```python
from build123d import *

# Parameters (mm, degrees)
EXTRUDE_1_DEPTH     = 43
SKETCH_2_R          = 1.65
CUT_EXTRUDE_1_DEPTH = 40
EXTRUDE_2_DEPTH     = 43
SKETCH_4_R          = 3.5
CUT_EXTRUDE_2_DEPTH = 15


with BuildPart() as part:
    # 草图1 → 凸台-拉伸1 (new body)
    with BuildSketch(Plane.XY):
        Polygon((0, 0), (7.053079228, 40), (37.053079228, 40), align=None)
    extrude(amount=EXTRUDE_1_DEPTH)

    # 草图2 → 切除-拉伸1 (cut)
    with BuildSketch(Plane(origin=(0, 40, 0), x_dir=(1, 0, 0), z_dir=(0, 1, 0))):
        with Locations(Location((10.053079228, -17, 0), (0, 0, 180))):
            Circle(SKETCH_2_R)
        with Locations(Location((10.053079228, -37, 0), (0, 0, 180))):
            Circle(SKETCH_2_R)
    extrude(amount=-CUT_EXTRUDE_1_DEPTH, mode=Mode.SUBTRACT)

    # 草图3 → 凸台-拉伸2 (add)
    with BuildSketch(Plane.XY.offset(43)):
        Polygon((2.644904711, 15), (-3.355095289, 15), (-3.355095289, 0), (0, 0), align=None)
    extrude(amount=-EXTRUDE_2_DEPTH)

    # 草图4 → 切除-拉伸2 (cut)
    with BuildSketch(Plane.XZ):
        with Locations(Location((10.053079228, 37, 0), (0, 0, 270))):
            Circle(SKETCH_4_R)
        with Locations(Location((10.053079228, 17, 0), (0, 0, 270))):
            Circle(SKETCH_4_R)
    extrude(amount=-CUT_EXTRUDE_2_DEPTH, mode=Mode.SUBTRACT)


solid = part.part
```
Work out the finished part from the listing and answer in its coordinate system (mm). A direction names the side the tool comes from. Coordinates: 2 decimals unless noted, no trailing zeros. Write each loop counter-clockwise with the first axis right and the second up, starting at its lowest first coordinate (ties: lowest second). Pieces come first, ordered by that corner, then holes.
Q1. A cutting plane is placed at A-A, the plane z = 17. Give the vertices of the cut face in (x, y).
Q2. Each of these flat-tipped pins is pushed along its axis until it touches: pin 1 Ø10 at (y, z) = (15, 9) entering from +X; pin 2 Ø8 at (x, z) = (10.05, 37) entering from -Y; pin 3 Ø5.5 at (x, z) = (10.05, 37) entering from -Y. Where does it stop, or does it pass through?
Q3. Which of the six approach directions +Z, -Z, +X, -X, +Y, -Y give full straight-line access (tool end or side, diameter ignored) to faces 4 (the face through (18.786, 20.28, 21.199)), 5 (the face through (6.636, 11.827, 17.759))?
Q4. A cutting plane is placed at D-D, the plane x = -1. Give the vertices of the cut face in (y, z), then the cut area to 3 significant figures.
Q5. Determine the mould class of faces 1 (the face through (0, 15, 22)), 2 (the face through (9, 15, 15)), 3 (the face through (4.82, 27.33, 21.2)) for opening direction X: released by +X, released by -X, zero draft, split by the parting line, or undercut.
Q6. A cutting plane is placed at C-C, the plane z = 12. Give the vertices of the cut face in (x, y), then the cut area to 3 significant figures.
Q7. Find the intervals of material crossed by line 1 (Z direction, x = 8, y = 11); line 2 (X direction, y = 34.5, z = 16); line 3 (X direction, y = 14.5, z = 32.5), in increasing order.
Q8. A cutting plane is placed at B-B, the plane y = 17.5. Give the vertices of the cut face in (x, z), then the cut area to 3 significant figures.
Findings below:
1. outline: (-3.36, 0) - (0, 0) - (6.55, 7.07) - (6.55, 15) - (8.4, 15) - (8.4, 40) - (7.05, 40) - (2.64, 15) - (-3.36, 15) - close; (11.7, 15) - (13.55, 15) - (13.55, 14.63) - (37.05, 40) - (11.7, 40) - close
2. pin 1: stops at x = 18.53
2. pin 2: stops at y = 6.53
2. pin 3: stops at y = 15
3. face 4: +Z, -Z, +X, -Y
3. face 5: -Y
4. outline: (0, 0) - (15, 0) - (15, 43) - (0, 43) - close
4. area: 645 mm2
5. face 1: zero draft
5. face 2: undercut
5. face 3: released by -X
6. outline: (-3.36, 0) - (0, 0) - (37.05, 40) - (7.05, 40) - (2.64, 15) - (-3.36, 15) - close
6. area: 670 mm2
7. line 1: z = 0 to 14.17, 19.83 to 34.17, 39.83 to 43
7. line 2: x = 6.08 to 8.74, 11.37 to 31.96
7. line 3: x = -3.36 to 13.43
8. outline: (3.09, 0) - (16.21, 0) - (16.21, 43) - (3.09, 43) - close; hole circle Ø3.3 at (10.05, 17); hole circle Ø3.3 at (10.05, 37)
8. area: 547 mm2
